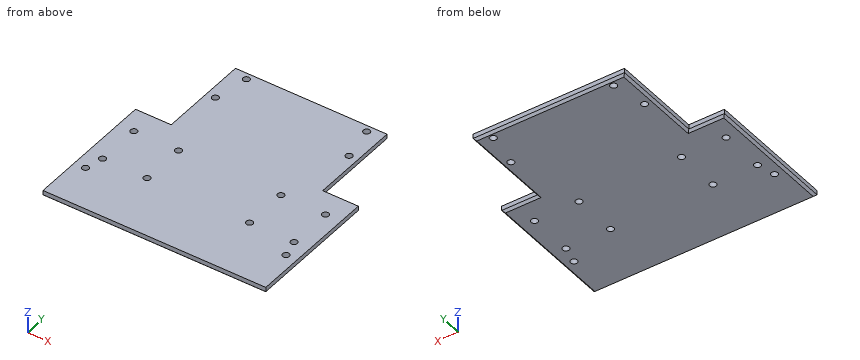
```python
from build123d import *

# Parameters (mm, degrees)
F0_W     = 100
F0_H     = 100
F1_DEPTH = 3
F3_D     = 3
F4_W     = 16
F4_H     = 41
F5_DEPTH = 3
F7_D     = 3
F8_SIZE  = 1
F10_D    = 3


with BuildPart() as f1:
    # F0 (on Top) → F1 (new body)
    with BuildSketch(Plane.XY):
        Rectangle(F0_W, F0_H)
    extrude(amount=F1_DEPTH)

    # F3 (through all)
    with Locations(Plane.XY.offset(3)):
        with Locations((-30, 31.5), (30, 31.5)):
            Hole(F3_D / 2)

    # F4 (on face) → F5 (cut)
    with BuildSketch(Plane.XY.offset(3)):
        with Locations((-42, 29.5)):
            Rectangle(F4_W, F4_H)
        with Locations((42, 29.5)):
            Rectangle(F4_W, F4_H)
    extrude(amount=-F5_DEPTH, mode=Mode.SUBTRACT)

    # F7 (through all)
    with Locations(Plane.XY.offset(3)):
        with Locations((-43, -2), (-23, -2), (-23, -22), (-43, -22), (23, -2), (43, -2), (43, -22), (23, -22)):
            Hole(F7_D / 2)

    # F8
    f8_edges = [f1.edges().sort_by_distance(p)[0] for p in [
        (0, -50, 0),
        (-50, -20.5, 0),
        (-42, 9, 0),
        (-34, 29.5, 0),
        (0, 50, 0),
        (34, 29.5, 0),
        (42, 9, 0),
        (50, -20.5, 0),
    ]]
    chamfer(f8_edges, length=F8_SIZE)

    # F10 (through all)
    with Locations(Plane.XY.offset(3)):
        with Locations((-45, -30), (45, -30), (-27, 47), (27, 47)):
            Hole(F10_D / 2)


solid = f1.part
```
Input: part model. Units: mm. Frame: model coordinates. Coordinates: 2 decimals unless noted, no trailing zeros. Loops run counter-clockwise (first coordinate to the right, second up) from the corner with the lowest first, then second, coordinate; pieces in that order, holes last. Notation, with made-up numbers: (30, 79) -> (74, 79) arc R20 ccw to (74, 114) -> close; hole circle Ø8 at (-33.5, 21). An arc over 180 degrees is marked (long way). Use a Markdown table: item, result.
1) Cut plane D-D (y = 31.5). Return the cut outline in (x, z), then the cut area to 3 significant figures.
Results found:
| item | result |
|---|---|
| outline | (-34, 1) -> (-33, 0) -> (-31.5, 0) -> (-31.5, 3) -> (-34, 3) -> close; (-28.5, 0) -> (28.5, 0) -> (28.5, 3) -> (-28.5, 3) -> close; (31.5, 0) -> (33, 0) -> (34, 1) -> (34, 3) -> (31.5, 3) -> close |
| area | 185 mm2 |
2) Cut plane C-C (x = -23). Return the cut outline in (y, z).
Results found:
| item | result |
|---|---|
| outline | (-50, 1) -> (-49, 0) -> (-23.5, 0) -> (-23.5, 3) -> (-50, 3) -> close; (-20.5, 0) -> (-3.5, 0) -> (-3.5, 3) -> (-20.5, 3) -> close; (-0.5, 0) -> (49, 0) -> (50, 1) -> (50, 3) -> (-0.5, 3) -> close |
3) Material intervals for line 1 along Y through (x, z) = (43, 2.2); line 2 along Y through (x, z) = (-23, 1.2); line 3 along Y through (x, z) = (27, 2.1), sorted ascending. Write a range as from..to.
Results found:
| item | result |
|---|---|
| line 1 | y = -50..-23.5, -20.5..-3.5, -0.5..9 |
| line 2 | y = -50..-23.5, -20.5..-3.5, -0.5..50 |
| line 3 | y = -50..45.5, 48.5..50 |
4) Cut plane B-B (y = -22). Return the cut outline in (x, z).
Results found:
| item | result |
|---|---|
| outline | (-50, 1) -> (-49, 0) -> (-44.5, 0) -> (-44.5, 3) -> (-50, 3) -> close; (-41.5, 0) -> (-24.5, 0) -> (-24.5, 3) -> (-41.5, 3) -> close; (-21.5, 0) -> (21.5, 0) -> (21.5, 3) -> (-21.5, 3) -> close; (24.5, 0) -> (41.5, 0) -> (41.5, 3) -> (24.5, 3) -> close; (44.5, 0) -> (49, 0) -> (50, 1) -> (50, 3) -> (44.5, 3) -> close |
5) Contact query for flat-ended pins moving along their axis: pin 1 (2.5 mm diameter, centred on x = -27, y = 47, fed in from -Z); pin 2 (3.5 mm diameter, centred on x = 43, y = -2, fed in from -Z); pin 3 (1.5 mm diameter, centred on y = 17.5, z = 0.5, fed in from -X); pin 4 (1.6 mm diameter, centred on x = -40, z = 2, fed in from +Y). Output: stop coordinate, or through.
Results found:
| item | result |
|---|---|
| pin 1 | passes through |
| pin 2 | stops at z = 0 |
| pin 3 | stops at x = -34 |
| pin 4 | stops at y = 9 |
6) Cut plane A-A (x = 27). Return the cut outline in (y, z), then the cut area to 3 significant figures.
Results found:
| item | result |
|---|---|
| outline | (-50, 1) -> (-49, 0) -> (45.5, 0) -> (45.5, 3) -> (-50, 3) -> close; (48.5, 0) -> (49, 0) -> (50, 1) -> (50, 3) -> (48.5, 3) -> close |
| area | 290 mm2 |
